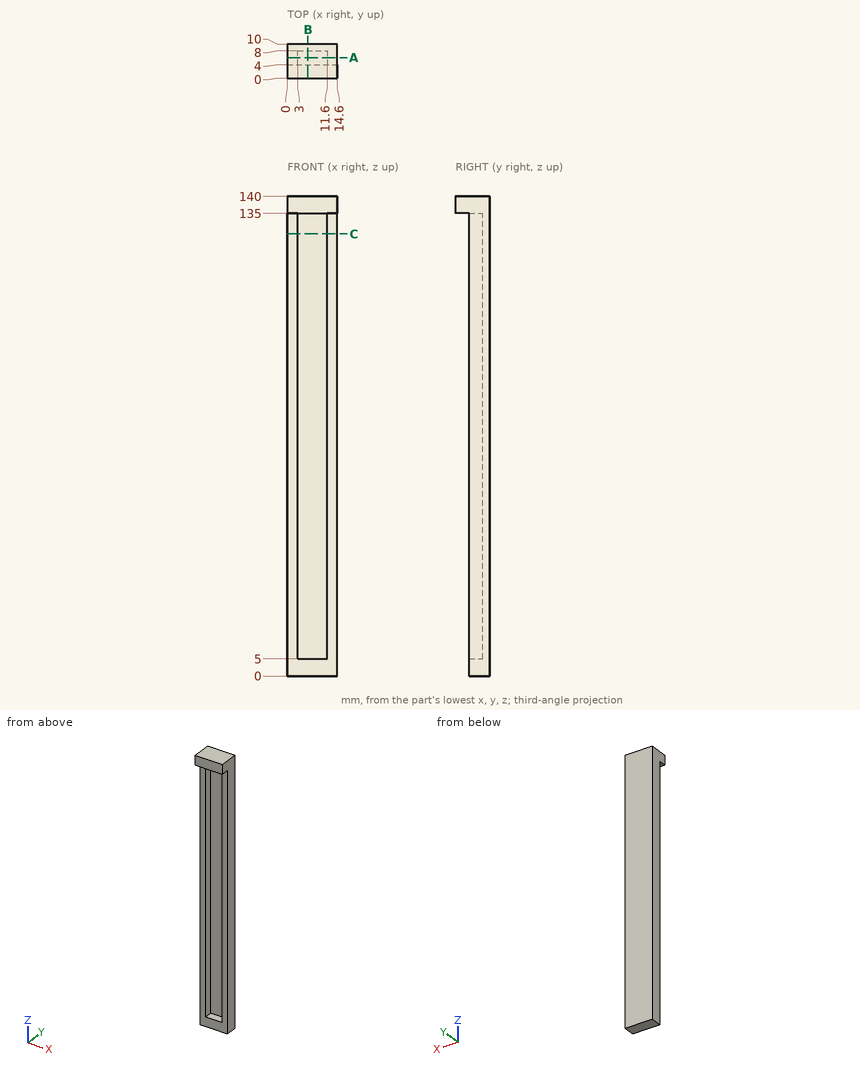
Geometry check sheet. Reference: drawing and pictorial views, mm from the part's lowest x, y, z. Round coordinates to 2 decimals unless told otherwise and drop trailing zeros. Loops run counter-clockwise (first coordinate to the right, second up) from the corner with the lowest first, then second, coordinate; pieces in that order, holes last. Notation, with made-up numbers: M 3,76.25 L 50,76.25 A19 ccw 50,112.25 Z; hole C 28,21.5 d8. An arc over 180 degrees is marked long. Return JSON: item names as keys, results as strings. Group by question number.
(1) Go/stop test with a flat-tipped pin: pin 1 (7.5 mm diameter, centred on x = 10.5, z = 94, fed in from -Y). Record where the tip stops, or that it passes through.
(2) Section check C-C, the plane z = 129. Enter the section's corners in (x, y), and give its area (3 significant figures).
(3) Section check A-A, the plane y = 6. Enter the section's corners in (x, z), and give its area (3 significant figures).
(4) Scan lines: line 1 along X through (y, z) = (4.5, 13); line 2 along Z through (x, y) = (7.75, 4.5); line 3 along Y through (x, z) = (11.5, 87.5). Record each from-to range of solid material in increasing order. Write a range as [from, to].
(5) Section check B-B, the plane x = 6. Enter the section's corners in (y, z), and give its area (3 significant figures).
Data:
{
 "1": {"pin 1": "y = 4"},
 "2": {"outline": "M 0,4 L 3,4 L 3,8 L 11.6,8 L 11.6,4 L 14.6,4 L 14.6,10 L 0,10 Z", "area": "53.2 mm²"},
 "3": {"outline": "M 0,0 L 14.6,0 L 14.6,140 L 0,140 Z; hole M 3,5 L 11.6,5 L 11.6,135 L 3,135 Z", "area": "926 mm²"},
 "4": {"line 1": "[0, 3], [11.6, 14.6]", "line 2": "[0, 5], [135, 140]", "line 3": "[8, 10]"},
 "5": {"outline": "M 0,135 L 8,135 L 8,5 L 4,5 L 4,0 L 10,0 L 10,140 L 0,140 Z", "area": "340 mm²"}
}
